```python
from build123d import *

# Parameters (mm, degrees)
F1_DEPTH  = 8
F2_D      = 5
F3_D      = 5
F5_DEPTH  = 7.5
F7_W      = 80
F7_H      = 8
F8_DEPTH  = 7
F9_W      = 80
F9_H      = 30
F10_DEPTH = 9


with BuildPart() as f1:
    # F0 (on Top) → F1 (new body)
    with BuildSketch(Plane.XY):
        with BuildLine():
            Line((40, -40), (40, 40))
            Line((40, 40), (10, 40))
            Line((10, 40), (10, 22))
            ThreePointArc((10, 22), (0, 12), (-10, 22))
            Line((-10, 22), (-10, 40))
            Line((-10, 40), (-40, 40))
            Line((-40, 40), (-40, -40))
            Line((-40, -40), (40, -40))
        make_face()
    extrude(amount=F1_DEPTH)

    # F2 (through all)
    with Locations(Plane(origin=(0, 0, 0), x_dir=(1, 0, 0), z_dir=(0, 0, -1))):
        with Locations((25.05, -22)):
            Hole(F2_D / 2)

    # F3 (through all)
    with Locations(Plane(origin=(0, 0, 0), x_dir=(1, 0, 0), z_dir=(0, 0, -1))):
        with Locations((-25.05, -22)):
            Hole(F3_D / 2)


with BuildPart() as f5:
    # F4 (on face) → F5 (new body, symmetric)
    with BuildSketch(Plane.XY.offset(8)):
        Polygon((-17.4625, 18), (-13.9983983849, 20), (-13.9983983849, 24), (-17.4625, 26), (-20.9266016151, 24), (-20.9266016151, 20), align=None)
    extrude(amount=F5_DEPTH, both=True)


with BuildPart() as f5b:
    # F4 (on face) → F5, piece 2 (new body, symmetric)
    with BuildSketch(Plane.XY.offset(8)):
        Polygon((17.4625, 18), (20.9266016151, 20), (20.9266016151, 24), (17.4625, 26), (13.9983983849, 24), (13.9983983849, 20), align=None)
    extrude(amount=F5_DEPTH, both=True)


with BuildPart() as f1_1:
    add(f1.part)

    # F6: cut F5, F5b
    add(f5.part, mode=Mode.SUBTRACT)
    add(f5b.part, mode=Mode.SUBTRACT)

    # F7 (on face) → F8 (join)
    with BuildSketch(Plane.XY):
        with Locations((-0.2263514698, -14)):
            Rectangle(F7_W, F7_H)
    extrude(amount=-F8_DEPTH)

    # F9 (on face) → F10 (join)
    with BuildSketch(Plane(origin=(0, 0, -7), x_dir=(1, 0, 0), z_dir=(0, 0, -1))):
        with Locations((-0.2263514698, 25)):
            Rectangle(F9_W, F9_H)
    extrude(amount=F10_DEPTH)


solid = f1_1.part
```
Source: CAD feature listing. Evaluate the final solid. Frame: model axes, mm. A direction names the side the tool comes from. Coordinates: 2 decimals unless noted, no trailing zeros. Write each loop counter-clockwise with the first axis right and the second up, starting at its lowest first coordinate (ties: lowest second). Pieces come first, ordered by that corner, then holes. Notation, with made-up numbers: (17, 13.25) - (56, 13.25) arc R31 cw to (56, 45.25) - close; hole circle Ø4 at (62.5, 84). An arc over 180 degrees is marked (long way). Answer as a JSON object with one key per item and string values.
Q1. Section query C-C, the plane z = 5.5. Output: boundary loops of the cut face in (x, y), plus the area to 3 significant figures.
Ans:
{"outline": "(-40, -40) - (40, -40) - (40, 40) - (10, 40) - (10, 22) arc R10 cw to (-10, 22) - (-10, 40) - (-40, 40) - close; hole circle Ø5 at (-25.05, 22); hole (-20.93, 20) - (-17.46, 18) - (-14, 20) - (-14, 24) - (-17.46, 26) - (-20.93, 24) - close; hole (14, 20) - (17.46, 18) - (20.93, 20) - (20.93, 24) - (17.46, 26) - (14, 24) - close; hole circle Ø5 at (25.05, 22)", "area": "5,760 mm2"}
Q2. Section query B-B, the plane x = -25.05. Output: boundary loops of the cut face in (y, z), plus the area to 3 significant figures.
Ans:
{"outline": "(-40, -16) - (-10, -16) - (-10, 0) - (19.5, 0) - (19.5, 8) - (-40, 8) - (-40, 0) - (-18, 0) - (-18, -7) - (-40, -7) - close; (24.5, 0) - (40, 0) - (40, 8) - (24.5, 8) - close", "area": "926 mm2"}
Q3. Section query D-D, the plane x = -8. Output: boundary loops of the cut face in (y, z), plus the area to 3 significant figures.
Ans:
{"outline": "(-40, -16) - (-10, -16) - (-10, 0) - (16, 0) - (16, 8) - (-40, 8) - (-40, 0) - (-18, 0) - (-18, -7) - (-40, -7) - close", "area": "774 mm2"}
Q4. Set-up query: faces 5 (the flat face through (-40, 1, 4)), 6 (the cylindrical face through (-24.72, 19.52, 4.06)), 7 (the flat face through (13.998, 22, 4)), 8 (the flat face through (39.774, -21, -10)). Return all of +Z, -Z, +X, -X, +Y, -Y with unobstructed straight access to the full face (end or side cutting, diameter ignored); none if empty.
Ans:
{"face 5": "+Z, -X, +Y, -Y", "face 6": "+Z, -Z", "face 7": "+Z", "face 8": "-Z, +X, +Y, -Y"}
Q5. Section query A-A, the plane y = -29. Output: boundary loops of the cut face in (x, z), plus the area to 3 significant figures.
Ans:
{"outline": "(-40.23, -16) - (39.77, -16) - (39.77, -7) - (-40.23, -7) - close; (-40, 0) - (40, 0) - (40, 8) - (-40, 8) - close", "area": "1,360 mm2"}
Q6. Material intervals for line 1 (X direction, y = 22, z = 5.5); line 2 (Y direction, x = -25.05, z = 6.5); line 3 (Z direction, x = 28.5, y = -24), sorted ascending. Write a range as [from, to].
Ans:
{"line 1": "x = [-40, -27.55], [-22.55, -20.93], [-14, -10], [10, 14], [20.93, 22.55], [27.55, 40]", "line 2": "y = [-40, 19.5], [24.5, 40]", "line 3": "z = [-16, -7], [0, 8]"}
Q7. First-contact query: pin 1 Ø9 at (y, z) = (-3.5, 5.5) entering from -X; pin 2 Ø8 at (y, z) = (-26, -7) entering from +X; pin 3 Ø3 at (x, z) = (30, -9) entering from +Y. Flat tips, straight axial feed; report the tip coordinate or a pass-through.
Ans:
{"pin 1": "stops at x = -40", "pin 2": "stops at x = 39.77", "pin 3": "stops at y = -10"}
Q8. Draft query along Y for faces 1 (the flat face through (40, -1, 4)), 2 (the flat face through (-19.219, 19.014, 4.302)), 3 (the cylindrical face through (0, 12, 4)), 4 (the flat face through (19.17, 18.986, 4.302)). Return one class per face: released by +Y, released by -Y, zero draft, split by the parting line, or undercut.
Ans:
{"face 1": "zero draft", "face 2": "undercut", "face 3": "released by +Y", "face 4": "undercut"}
